Here's how the part is built. I have some questions about the finished solid (model axes, mm). A direction names the side the tool comes from. Round coordinates to 2 decimals unless told otherwise and drop trailing zeros. Loops run counter-clockwise (first coordinate to the right, second up) from the corner with the lowest first, then second, coordinate; pieces in that order, holes last. Notation, with made-up numbers: M -16,-1.5 L 39,-1.5 A27 ccw 39,18.5 Z; hole C -10,42 d9. An arc over 180 degrees is marked long. Answer as a JSON object with one key per item and string values.
Autodesk Inventor part; units mm, degrees
ref_plane "Start plane" through (0, 0, -20) normal (0, 0, 1) x (1, 0, 0)
ref_plane "End plane" through (0, 0, 1520) normal (0, 0, 1) x (1, 0, 0)
ref_plane "Work Plane4" through (20, 0, -20) normal (-0.7071, 0, -0.7071) x (-0.7071, 0, 0.7071)
ref_plane "Start plane" through (0, 0, -20) normal (0, 0, 1) x (1, 0, 0)
ref_plane "End plane" through (0, 0, 1520) normal (0, 0, 1) x (1, 0, 0)
sketch "Sketch" plane through (0, 0, 0) normal (0, 0, 1) x (1, 0, 0)
  line L0 (-20, -12) -> (-20, 12)
  line L1 (-12, 20) -> (12, 20)
  line L2 (20, 12) -> (20, -12)
  line L3 (12, -20) -> (-12, -20)
  arc A0 (-20, -12) -> (-12, -20) centre (-12, -12) ccw
  arc A1 (-12, 20) -> (-20, 12) centre (-12, 12) ccw
  arc A2 (20, 12) -> (12, 20) centre (12, 12) ccw
  arc A3 (12, -20) -> (20, -12) centre (12, -12) ccw
  arc A4 (-12, 16) -> (-16, 12) centre (-12, 12) ccw
  line L4 (-12, 16) -> (12, 16)
  arc A5 (16, 12) -> (12, 16) centre (12, 12) ccw
  line L5 (16, 12) -> (16, -12)
  arc A6 (12, -16) -> (16, -12) centre (12, -12) ccw
  line L6 (12, -16) -> (-12, -16)
  arc A7 (-16, -12) -> (-12, -16) centre (-12, -12) ccw
  line L7 (-16, -12) -> (-16, 12)
  line L8 (0, 30.3196) -> (0, -30.3196) construction
  line L9 (-30.3196, 0) -> (30.3196, 0) construction
  dimension "d7" = 8
  dimension "d10" = 40
  dimension "d11" = 40
  dimension "d12" = 4
  dimension "d15" = 20
  dimension "d16" = 20
extrude "Body" add sketch "Sketch" along normal up to surface (1540 mm away) from surface at -20
sketch "Sketch3" plane through (0, 0, 0) normal (0, 0, 1) x (1, 0, 0)
  line L0 (0, 0) -> (10, 0)
ref_plane "Work Plane3" through (0, 0, 0) normal (0, -1, 0) x (1, 0, 0)
sketch "Sketch4" plane through (0, 0, 0) normal (0, -1, 0) x (1, 0, 0)
  line L0 (-2, -20) -> (12, -20)
  line L1 (-2, 1520) -> (12, 1520)
  dimension "d18" = 1540
ref_plane "Work Plane4" through (20, 0, -20) normal (-0.7071, 0, -0.7071) x (-0.7071, 0, 0.7071)
split "Split1" plane through (20, 0, -20) removes the side toward (-0.7071, 0, -0.7071)
ref_plane "Work Plane5" through (20, 0, 1520) normal (-0.7071, 0, 0.7071) x (0.7071, 0, 0.7071)
split "Split2" plane through (20, 0, 1520) removes the side toward (-0.7071, 0, 0.7071)
equation "\"d7\" = G_IR"
equation "\"d10\" = G_H"
equation "\"d11\" = G_W"
equation "\"d12\" = G_T"
equation "\"d15\" = 0.5 * d10"
equation "\"d16\" = 0.5 * d11"
equation "\"d3\" = G_L"
equation "\"G_W\" = 40"
equation "\"G_H\" = 40"
equation "\"G_T\" = 4"
equation "\"G_IR\" = 8"
equation "\"G_L\" = d18"
equation "\"G_OFFSET_START\" = 20"
equation "\"G_OFFSET_END\" = 20"
equation "\"d13\" = -G_OFFSET_START"
equation "\"d14\" = G_OFFSET_END + B_L"
properties part number "DIN EN 10219-2 - 40 x 40 x 4  - 1540" material "Steel, Mild"
Item 1: We'd pull the mould along X, two halves only. Please class faces 3 (the face through (20, 0, 739)), 4 (the face through (0, 16, 739)), 5 (the face through (-0.1, -16.4, 1499.9)): +X half, -X half, draft (parallel to the pull), parting line (faces both ways), or undercut.
Solution:
{"face 3": "+X half", "face 4": "undercut", "face 5": "-X half"}
Item 2: I want a section at B-B on x = 1. List the corners of the cut face in (y, z) for me, plus the area to 3 significant figures.
Solution:
{"outline": "M -20,-1 L -16,-1 L -16,1501 L -20,1501 Z; M 16,-1 L 20,-1 L 20,1501 L 16,1501 Z", "area": "12,000 mm2"}
Item 3: For faces 1 (the face through (0, -16, 739)), 2 (the face through (0, -20, 739)), which set-ups out of +Z, -Z, +X, -X, +Y, -Y let a thin tool reach every point of the face, with its end or its side?
Solution:
{"face 1": "+Z, -Z", "face 2": "+Z, -Z, +X, -X, -Y"}
Item 4: I want a section at C-C on y = -2. List the corners of the cut face in (x, z) for me, plus the area to 3 significant figures.
Solution:
{"outline": "M -20,20 L -16,16 L -16,1484 L -20,1480 Z; M 16,-16 L 20,-20 L 20,1520 L 16,1516 Z", "area": "12,000 mm2"}
Item 5: For P1, Ø5, axis at x = 6, y = 11.5, coming from the -Z side, with a flat end and sliding along its axis, tell me the tip position at first contact or that it passes through.
Solution:
{"P1": "passes through"}
Item 6: If I drill on L1, parallel to Y at x = 9.5, z = 1455.5; L2, parallel to X at y = 13, z = 1138, over which ranges is the centre line in solid material (lowest first)? Write a range as from..to.
Solution:
{"L1": "y = -20..-16, 16..20", "L2": "x = -19.94..-15.87, 15.87..19.94"}
Item 7: I want a section at A-A on z = 75.5. List the corners of the cut face in (x, y) for me.
Solution:
{"outline": "M -20,-12 A8 ccw -12,-20 L 12,-20 A8 ccw 20,-12 L 20,12 A8 ccw 12,20 L -12,20 A8 ccw -20,12 Z; hole M -16,-12 A4 ccw -12,-16 L 12,-16 A4 ccw 16,-12 L 16,12 A4 ccw 12,16 L -12,16 A4 ccw -16,12 Z"}
